```python
from build123d import *

# Parameters (mm, degrees)
BOSS_EXTRUDE1_DEPTH   = 11
BOSS_EXTRUDE1_2_DEPTH = 11
SKETCH2_W             = 5.7
SKETCH2_H             = 6
CUT_EXTRUDE1_DEPTH    = 3
BOSS_EXTRUDE8_DEPTH   = 11
BOSS_EXTRUDE2_DEPTH   = 6
BOSS_EXTRUDE3_START   = -5.5
BOSS_EXTRUDE3_DEPTH   = 2.5
FILLET7_R             = 1
FILLET8_R             = 1
FILLET10_R            = 1
FILLET11_R            = 1
FILLET12_R            = 0.5
BOSS_EXTRUDE7_REACH   = 36.321
BOSS_EXTRUDE7_START   = 5.5
SKETCH6_R             = 5.5
SKETCH6_R_2           = 4.5
CUT_EXTRUDE3_DEPTH    = 29.820825804
BOSS_EXTRUDE9_DEPTH   = 11


with BuildPart() as part:
    # Sketch1 → Boss-Extrude1 (new body)
    with BuildSketch(Plane.XY):
        Polygon((0, 3.8), (0, 2), (-10.5, 3.5), (-21.5, 3.5), (-23, 4), (-24.5, 3.5), (-26, 3.5), (-26, 5.3), (-24.5, 5.3), (-23, 5.8), (-21.5, 5.3), (-10.5, 5.3), align=None)
    extrude(amount=BOSS_EXTRUDE1_DEPTH)



with BuildPart() as body_2:
    # Sketch1 → Boss-Extrude1 2 (new body)
    with BuildSketch(Plane.XY):
        Polygon((0, 0), (0, -2.5), (-26, -2.5), (-26, 0), (-24.5, 0), (-23, -0.5), (-21.5, 0), align=None)
    extrude(amount=BOSS_EXTRUDE1_2_DEPTH)

    # Sketch2 → Cut-Extrude1 (cut)
    with BuildSketch(Plane.XZ.offset(2.5)):
        with Locations((-18.55, 5.5)):
            Rectangle(SKETCH2_W, SKETCH2_H)
    extrude(amount=-CUT_EXTRUDE1_DEPTH, mode=Mode.SUBTRACT)


with BuildPart() as part_1:
    add(part.part)

    add(body_2.part)  # Boss-Extrude8 merges body 2
    # Sketch8 → Boss-Extrude8 (add)
    with BuildSketch(Plane(origin=(0, 0, 0), x_dir=(-1, 0, 0), z_dir=(0, 0, -1))):
        with BuildLine():
            Line((0.948237354, 2.135462479), (0, 2))
            Line((0, 2), (0, 0))
            Line((0, 0), (1.1, 0))
            ThreePointArc((1.1, 0), (0.029575797, 0.997051253), (0.948237354, 2.135462479))
        make_face()
    extrude(amount=-BOSS_EXTRUDE8_DEPTH)

    # Sketch3 → Boss-Extrude2 (add)
    with BuildSketch(Plane.XY.offset(2.5)):
        Polygon((-15.7, 0), (-17.7, -2), (-17.7, -2.5), (-15.7, -2.5), align=None)
    extrude(amount=BOSS_EXTRUDE2_DEPTH)

    # Sketch4 → Boss-Extrude3 (add, symmetric)
    with BuildSketch(Plane.XY.offset(11).offset(BOSS_EXTRUDE3_START)):
        with BuildLine():
            Line((-18.9, -2), (-16.9, 0))
            Line((-16.9, 0), (-16.9, 0.4))
            Line((-16.9, 0.4), (-18.4, 0.4))
            Line((-18.4, 0.4), (-18.4, 1.9))
            ThreePointArc((-18.4, 1.9), (-17.93137085, 3.03137085), (-16.8, 3.5))
            Line((-16.8, 3.5), (-20.3, 3.5))
            Line((-20.3, 3.5), (-20.3, -3))
            Line((-20.3, -3), (-18.9, -3))
            Line((-18.9, -3), (-18.9, -2))
        make_face()
    extrude(amount=BOSS_EXTRUDE3_DEPTH, both=True)

    # Fillet7
    fillet7_edges = [part_1.edges().sort_by_distance(p)[0] for p in [
        (-26, 0, 5.5),
    ]]
    fillet(fillet7_edges, radius=FILLET7_R)

    # Fillet8
    fillet8_edges = [part_1.edges().sort_by_distance(p)[0] for p in [
        (-26, 3.5, 5.5),
    ]]
    fillet(fillet8_edges, radius=FILLET8_R)

    # Fillet10
    # the kernel refuses this fillet: 1 mm, written as the material it takes off along each edge
    with BuildSketch(Plane(origin=(-26, 5.3, -2.449489743), x_dir=(1.6120438317551944e-12, -1.0, 0), z_dir=(0, 0, 1))) as fillet10_piece_1:
        with BuildLine():
            CenterArc((1, 0.979795897), FILLET10_R, 180, 78.463040967)
            Line((0, 0.979795897), (-0.02, 0.979795897))
            Line((-0.02, 0.979795897), (-0.02, 0))
            Line((-0.02, 0), (0, -0.02))
            ThreePointArc((0, -0.02), (0.4, -0.02), (0.796, -0.019595918))
            Line((0.796, -0.019595918), (0.8, 0))
        make_face()
    extrude(amount=15.898979486, mode=Mode.SUBTRACT)

    # Fillet11
    fillet11_edges = [part_1.edges().sort_by_distance(p)[0] for p in [
        (-26, -2.5, 5.5),
    ]]
    fillet(fillet11_edges, radius=FILLET11_R)

    # Fillet12
    fillet12_edges = [part_1.edges().sort_by_distance(p)[0] for p in [
        (-18.9, -3, 5.5),
        (-20.3, -3, 5.5),
    ]]
    fillet(fillet12_edges, radius=FILLET12_R)

    # Sketch6 → Boss-Extrude7 (add, up to next)
    with BuildSketch(Plane(origin=(0, 0, 0), x_dir=(1, 0, 0), z_dir=(0, 1, 0)).offset(BOSS_EXTRUDE7_START), mode=Mode.PRIVATE) as boss_extrude7_sk1:
        with Locations(Location((-10.75, -5.5, 0), (0, 0, 270))):
            Circle(SKETCH6_R)
        with Locations(Location((-10.75, -5.5, 0), (0, 0, 270))):
            Circle(SKETCH6_R_2, mode=Mode.SUBTRACT)
    boss_extrude7_tool1 = extrude(boss_extrude7_sk1.sketch, amount=-BOSS_EXTRUDE7_REACH, mode=Mode.PRIVATE) - part_1.part
    add(boss_extrude7_tool1.solids().sort_by_distance((-10.75, 5.5, 0.155563))[0])

    # Sketch7 → Cut-Extrude3 (cut, through all)
    with BuildSketch(Plane.XY):
        Polygon((-10.5, 5.5), (-0.5, 4.071428571), (-0.5, 5.5), align=None)
    extrude(amount=CUT_EXTRUDE3_DEPTH, mode=Mode.SUBTRACT)

    # Sketch10 → Boss-Extrude9 (add)
    with BuildSketch(Plane(origin=(0, 0, 0), x_dir=(-1, 0, 0), z_dir=(0, 0, -1))):
        Polygon((0, -2.5), (4.936344802, -2.5), (0, -5.35), align=None)
    extrude(amount=-BOSS_EXTRUDE9_DEPTH)


solid = part_1.part
```
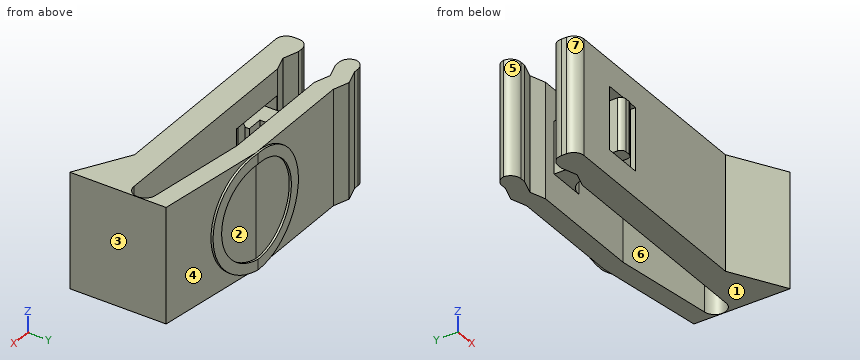
The listing builds one solid part. Answer for the finished solid, in the listing's coordinates (mm). Face numbers are marked on the shaded views. A direction names the side the tool comes from. Coordinates: 2 decimals unless noted, no trailing zeros. Loops run counter-clockwise (first coordinate to the right, second up) from the corner with the lowest first, then second, coordinate; pieces in that order, holes last. Notation, with made-up numbers: (82, 41) -> (114, 41) arc R17 ccw to (114, 69) -> close; hole circle Ø1 at (63.5, 40). An arc over 180 degrees is marked (long way). Return JSON: item names as keys, results as strings. Group by question number.
(1) Determine the mould class of the marked faces 1, 2 and 3 for opening direction Z: released by +Z, released by -Z, zero draft, split by the parting line, or undercut.
(2) A cutting plane is placed at D-D on x = -3.5. Write down the section's boundary in (y, z), and give its area (3 significant figures).
(3) Given pin 1 Ø4 at (x, z) = (-10.5, 4.5) entering from -Y; pin 2 Ø1.6 at (x, z) = (-17.5, 6.5) entering from +Y, each flat-ended and moving along its own axis, determine where each tip first touches the part or whether it passes through.
(4) A cutting plane is placed at B-B on y = 1.5. Write down the section's boundary in (x, z).
(5) Find the intervals of material crossed by probe 1 along Y at (x, z) = (-15, 9.75); probe 2 along Y at (x, z) = (-15.5, 3.25); probe 3 along X at (y, z) = (-0.75, 6), in increasing order. Write a range as from..to.
(6) A cutting plane is placed at A-A on x = -15. Write down the section's boundary in (y, z).
(7) Which of the six approach directions +Z, -Z, +X, -X, +Y, -Y give full straight-line access (tool end or side, diameter ignored) to the marked faces 4, 5, 6 and 7?
The answers:
{
 "1": {"face 1": "released by -Z", "face 2": "undercut", "face 3": "zero draft"},
 "2": {"outline": "(-3.33, 0) -> (0, 0) -> (0, 11) -> (-3.33, 11) -> close; (2.5, 0) -> (4.3, 0) -> (4.3, 11) -> (2.5, 11) -> close", "area": "56.4 mm^2"},
 "3": {"pin 1": "stops at y = -2.5", "pin 2": "stops at y = 5.3"},
 "4": {"outline": "(-20.3, 3) -> (-18.4, 3) -> (-18.4, 8) -> (-20.3, 8) -> close; (-0.12, 0) -> (0, 0) -> (0, 11) -> (-0.12, 11) -> close"},
 "5": {"probe 1": "y = -2.5..0, 3.5..5.3", "probe 2": "y = -2.5..0, 3.5..5.5", "probe 3": "x = -25.97..-21.4, -20.3..-17.65, -16.45..0"},
 "6": {"outline": "(-2.5, 0) -> (0, 0) -> (0, 11) -> (-2.5, 11) -> close; (3.5, 0) -> (5.3, 0) -> (5.3, 2.01) -> (5.5, 2.01) -> (5.5, 4.02) -> (5.3, 4.02) -> (5.3, 6.98) -> (5.5, 6.98) -> (5.5, 8.99) -> (5.3, 8.99) -> (5.3, 11) -> (3.5, 11) -> close"},
 "7": {"face 4": "+X, +Y", "face 5": "+Z, -Z, -X", "face 6": "+Z, -Z", "face 7": "+Z, -Z, -X, -Y"}
}
